from build123d import *

# Parameters (mm, degrees)
F0_W     = 256.54
F0_H     = 50.8
F1_DEPTH = 254
F2_T     = -1.27
F3_R     = 2.54


with BuildPart() as f1:
    # F0 (on Front) → F1 (new body)
    with BuildSketch(Plane.XZ):
        Rectangle(F0_W, F0_H)
    extrude(amount=F1_DEPTH)

    # F2
    f2_openings = [f1.faces().sort_by_distance(p)[0] for p in [
        (0, -254, 0),
        (0, -127, -25.4),
        (0, 0, 0),
    ]]
    offset(amount=F2_T, openings=f2_openings)

    # F3
    f3_edges = [f1.edges().sort_by_distance(p)[0] for p in [
        (-127, -127, 24.13),
        (127, -127, 24.13),
        (128.27, -127, 25.4),
        (-128.27, -127, 25.4),
    ]]
    fillet(f3_edges, radius=F3_R)


solid = f1.part
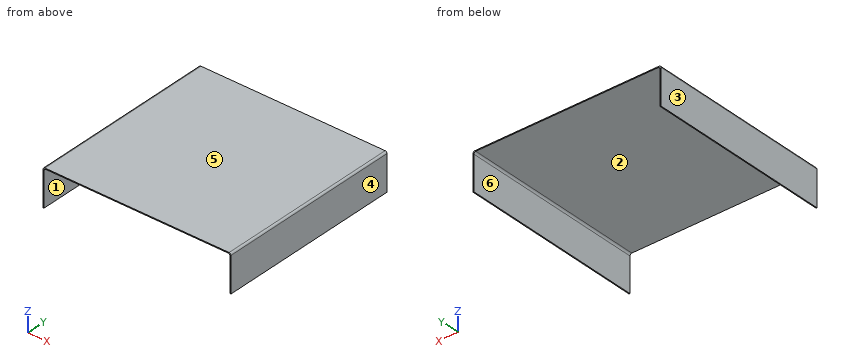
The listing builds one solid part. Answer for the finished solid, in the listing's coordinates (mm). Face numbers are marked on the shaded views. A direction names the side the tool comes from. Round coordinates to 2 decimals unless told otherwise and drop trailing zeros. Write each loop counter-clockwise with the first axis right and the second up, starting at its lowest first coordinate (ties: lowest second). Pieces come first, ordered by that corner, then holes. Notation, with made-up numbers: M 14.5,3.5 L 68.5,3.5 A26 ccw 68.5,19.5 Z; hole C -9.5,46 d3. An arc over 180 degrees is marked long. Write each question's results on one line, items separated by ' | '. Start each with the question number.
Item 1: Find section A-A on y = -166.5. Write down the section's boundary in (x, z), and give its area (3 significant figures).
Item 2: The mould has two halves that part along X. Classify the marked faces 1, 2, 3 and 4: +X half, -X half, draft (parallel to the pull), parting line (faces both ways), or undercut.
Item 3: Which of the six approach directions +Z, -Z, +X, -X, +Y, -Y give full straight-line access (tool end or side, diameter ignored) to the marked faces 5 and 6?
Item 4: Find section C-C on x = 77. Write down the section's boundary in (y, z), and give its area (3 significant figures).
Item 5: Find section B-B on z = 16. Write down the section's boundary in (x, y).
Item 6: Straight lines are drawn through the part: probe 1 along X at (y, z) = (-167, 21); probe 2 along Z at (x, y) = (-23, -107). For each, find the intervals that lie inside material, in ascending order.
Item 7: Given pin 1 Ø6 at (x, y) = (-76, -34) entering from -Z, flat-ended and moving along its own axis, determine where the tip first touches the part or whether it passes through.
Answer block:
1) outline: M -128.27,-25.4 L -127,-25.4 L -127,21.59 A2.54 cw -124.46,24.13 L 124.46,24.13 A2.54 cw 127,21.59 L 127,-25.4 L 128.27,-25.4 L 128.27,22.86 A2.54 ccw 125.73,25.4 L -125.73,25.4 A2.54 ccw -128.27,22.86 Z | area: 452 mm²
2) face 1: undercut | face 2: undercut | face 3: -X half | face 4: +X half
3) face 5: +Z, +X, -X, +Y, -Y | face 6: -Z, +Y, -Y
4) outline: M -254,24.13 L 0,24.13 L 0,25.4 L -254,25.4 Z | area: 323 mm²
5) outline: M -128.27,-254 L -127,-254 L -127,0 L -128.27,0 Z; M 127,-254 L 128.27,-254 L 128.27,0 L 127,0 Z
6) probe 1: x = -128.27 to -127, 127 to 128.27 | probe 2: z = 24.13 to 25.4
7) pin 1: stops at z = 24.13
